Geometry check sheet. Reference: the model listing, model coordinates, mm. A direction names the side the tool comes from. Coordinates: 2 decimals unless noted, no trailing zeros. Write each loop counter-clockwise with the first axis right and the second up, starting at its lowest first coordinate (ties: lowest second). Pieces come first, ordered by that corner, then holes. Notation, with made-up numbers: (-24, -6.75) -> (18, -6.75) arc R19 ccw to (18, 15.25) -> close; hole circle Ø5 at (47, 74). An arc over 180 degrees is marked (long way). Answer in a Markdown table with one row per item. Add a question column.
1. Set-up check for faces 4 (the flat face through (2, -200, -5)), 5 (the flat face through (-3, -205, 2)): record each of +Z, -Z, +X, -X, +Y, -Y from which the full face is reachable in a straight line by a thin tool's end or side.
2. Cross-section at A-A on x = -8. Record the cut outline in (y, z).
3. Cross-section at C-C on y = -127. Record the cut outline in (x, z), and give its area (3 significant figures).
4. Cross-section at B-B on z = 0. Record the cut outline in (x, y), and give its area (3 significant figures).
5. Depth check by flat-ended pin: P1, Ø8, axis at x = 119.5, z = -41, coming from the +Y side. Enter the tip coordinate at first touch or a pass-through.
6. Cross-section at D-D on x = -129. Record the cut outline in (y, z), and give its area (3 significant figures).
7. Mould release check, pull along Z, two halves, no side actions. Record for faces 1 (the flat face through (-180, -101, -2)), 2 (the flat face through (-3, -101, -150)), 3 (the cylindrical face through (177.465, -142.564, -0.976)): pulls with the +Z half, pulls with the -Z half, needs draft (parallel to the pull), parting line crosses it, or undercut.
8. Scan lines: L1, parallel to X at y = -3.15, z = 85; L2, parallel to Y at x = 40.5, z = -6; L3, parallel to X at y = -107, z = -46. Record each from-to range of solid material in increasing order. Write a range as from..to.
```python
from build123d import *

# Parameters (mm, degrees)
SKETCH1_W           = 360
SKETCH1_H           = 300
BOSS_EXTRUDE1_DEPTH = 200
SKETCH2_W           = 350
SKETCH2_H           = 290
CUT_EXTRUDE1_DEPTH  = 195
SKETCH3_W           = 30
SKETCH3_H           = 290
CUT_EXTRUDE2_DEPTH  = 309.058436015
SKETCH4_R           = 7.5
CUT_EXTRUDE3_DEPTH  = 439.292140016
SKETCH5_R           = 2.5
CUT_EXTRUDE4_DEPTH  = 5
SKETCH6_W           = 360
SKETCH6_H           = 300
BOSS_EXTRUDE2_DEPTH = 5
SKETCH7_W           = 200
SKETCH7_H           = 27
CUT_EXTRUDE5_DEPTH  = 5


with BuildPart() as part:
    # Sketch1 → Boss-Extrude1 (new body)
    with BuildSketch(Plane(origin=(0, 0, 0), x_dir=(1, 0, 0), z_dir=(0, 1, 0))):
        Rectangle(SKETCH1_W, SKETCH1_H)
    extrude(amount=-BOSS_EXTRUDE1_DEPTH)

    # Sketch2 → Cut-Extrude1 (cut)
    with BuildSketch(Plane.XZ.offset(200)):
        Rectangle(SKETCH2_W, SKETCH2_H)
    extrude(amount=-CUT_EXTRUDE1_DEPTH, mode=Mode.SUBTRACT)

    # Sketch3 → Cut-Extrude2 (cut, through all)
    with BuildSketch(Plane(origin=(0, 0, 0), x_dir=(1, 0, 0), z_dir=(0, 1, 0))):
        Rectangle(SKETCH3_W, SKETCH3_H)
    extrude(amount=-CUT_EXTRUDE2_DEPTH, mode=Mode.SUBTRACT)

    # Sketch4 → Cut-Extrude3 (cut, through all)
    with BuildSketch(Plane.ZY.offset(180)):
        with Locations((0, -150)):
            Circle(SKETCH4_R)
    extrude(amount=-CUT_EXTRUDE3_DEPTH, mode=Mode.SUBTRACT)

    # Sketch5 → Cut-Extrude4 (cut)
    with BuildSketch(Plane(origin=(0, 0, 0), x_dir=(1, 0, 0), z_dir=(0, 1, 0))):
        with Locations(Location((-25, 85, 0), (0, 0, 270))):
            Circle(SKETCH5_R)
        with Locations(Location((25, 85, 0), (0, 0, 270))):
            Circle(SKETCH5_R)
        with Locations(Location((25, -85, 0), (0, 0, 270))):
            Circle(SKETCH5_R)
        with Locations(Location((-25, -85, 0), (0, 0, 270))):
            Circle(SKETCH5_R)
    extrude(amount=-CUT_EXTRUDE4_DEPTH, mode=Mode.SUBTRACT)

    # Sketch6 → Boss-Extrude2 (add)
    with BuildSketch(Plane.XZ.offset(200)):
        Rectangle(SKETCH6_W, SKETCH6_H)
    extrude(amount=BOSS_EXTRUDE2_DEPTH)

    # Sketch7 → Cut-Extrude5 (cut)
    with BuildSketch(Plane(origin=(0, 0, -150), x_dir=(-1, 0, 0), z_dir=(0, 0, -1))):
        with Locations((0, -186.5)):
            Rectangle(SKETCH7_W, SKETCH7_H)
    extrude(amount=-CUT_EXTRUDE5_DEPTH, mode=Mode.SUBTRACT)


solid = part.part
```
Results found:
| question | item | result |
|---|---|---|
| 1 | face 4 | none |
| 1 | face 5 | +Z, -Z, +X, -X, -Y |
| 2 | outline | (-205, -150) -> (-200, -150) -> (-200, 145) -> (0, 145) -> (0, 150) -> (-205, 150) -> close; (-173, -150) -> (0, -150) -> (0, -145) -> (-173, -145) -> close |
| 3 | outline | (-180, -150) -> (180, -150) -> (180, 150) -> (-180, 150) -> close; hole (-175, -145) -> (175, -145) -> (175, 145) -> (-175, 145) -> close |
| 3 | area | 6,500 mm^2 |
| 4 | outline | (-180, -205) -> (180, -205) -> (180, -157.5) -> (175, -157.5) -> (175, -200) -> (-175, -200) -> (-175, -157.5) -> (-180, -157.5) -> close; (-180, -142.5) -> (-175, -142.5) -> (-175, -5) -> (-15, -5) -> (-15, 0) -> (-180, 0) -> close; (15, -5) -> (175, -5) -> (175, -142.5) -> (180, -142.5) -> (180, 0) -> (15, 0) -> close |
| 4 | area | 5,250 mm^2 |
| 5 | P1 | stops at y = 0 |
| 6 | outline | (-205, -150) -> (0, -150) -> (0, 150) -> (-205, 150) -> close; hole (-200, -145) -> (-5, -145) -> (-5, 145) -> (-200, 145) -> close |
| 6 | area | 4,950 mm^2 |
| 7 | face 1 | needs draft |
| 7 | face 2 | pulls with the -Z half |
| 7 | face 3 | undercut |
| 8 | L1 | x = -180..-27.5, -22.5..-15, 15..22.5, 27.5..180 |
| 8 | L2 | y = -205..-200, -5..0 |
| 8 | L3 | x = -180..-175, 175..180 |
